The listing builds one solid part. Answer for the finished solid, in the listing's coordinates (mm). Face numbers are marked on the shaded views. A direction names the side the tool comes from. Give positions to 0.01 mm unless a question says otherwise; leave off trailing zeros. Write each loop counter-clockwise with the first axis right and the second up, starting at its lowest first coordinate (ties: lowest second). Pieces come first, ordered by that corner, then holes. Notation, with made-up numbers: (77, 46.5) - (93, 46.5) arc R17 ccw to (93, 79.5) - close; hole circle Ø3 at (-34, -5). An arc over 180 degrees is marked (long way). One line per question, with ' | ' between items. Start each with the question number.
1. A cutting plane is placed at A-A (z = 3). Determine the outline of the cut face in (x, y).
2. A cutting plane is placed at C-C (y = 27.25). Determine the outline of the cut face in (x, z), then the cut area to 3 significant figures.
3. A cutting plane is placed at D-D (z = -6.25). Determine the outline of the cut face in (x, y).
4. For the marked faces 4 and 5, determine the directions among +Z, -Z, +X, -X, +Y, -Y from which every point of the face is accessible in a straight line to the end or side of a thin tool.
5. The mould has two halves that part along Y. Classify the marked faces 1, 2 and 3: +Y half, -Y half, draft (parallel to the pull), parting line (faces both ways), or undercut.
6. A cutting plane is placed at B-B (x = 7.5). Determine the outline of the cut face in (y, z), then the cut area to 3 significant figures.
7. Given P1, Ø8.5, axis at x = -3, y = 21.5, coming from the +Z side; P2, Ø4, axis at x = 7, z = 6, coming from the +Y side, each flat-ended and moving along its own axis, determine where each tip first touches the part or whether it passes through.
8. Find the intervals of material crossed by L1, parallel to Y at x = 0, z = -8.3; L2, parallel to Z at x = 5, y = 9.5; L3, parallel to Y at x = 10, z = -3, in increasing order. Write a range as from..to.
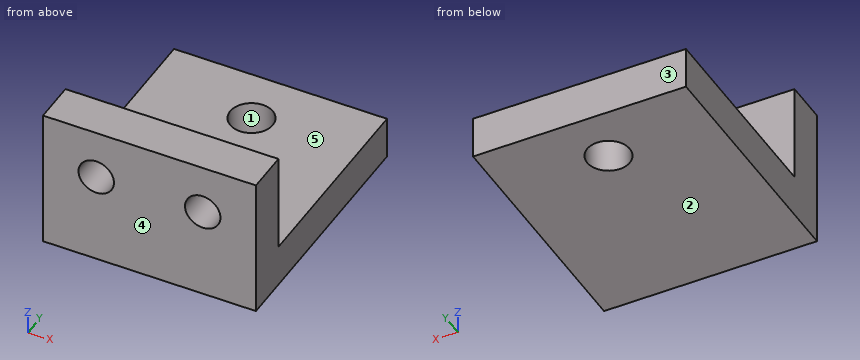
```python
from build123d import *

# Parameters (mm, degrees)
CROQUIS1_W              = 30
CROQUIS1_H              = 20
SALIENTE_EXTRUIR1_DEPTH = 6
CROQUIS2_W              = 30
CROQUIS2_H              = 35
SALIENTE_EXTRUIR2_DEPTH = 6
CROQUIS3_R              = 3
CORTAR_EXTRUIR1_DEPTH   = 6
CROQUIS4_R              = 2.5
CORTAR_EXTRUIR2_DEPTH   = 6


with BuildPart() as part:
    # Croquis1 → Saliente-Extruir1 (new body)
    with BuildSketch(Plane(origin=(0, 0, 0), x_dir=(1, 0, 0), z_dir=(0, 1, 0))):
        Rectangle(CROQUIS1_W, CROQUIS1_H)
    extrude(amount=SALIENTE_EXTRUIR1_DEPTH)

    # Croquis2 → Saliente-Extruir2 (add)
    with BuildSketch(Plane(origin=(0, 0, -10), x_dir=(-1, 0, 0), z_dir=(0, 0, -1))):
        with Locations((0, 17.5)):
            Rectangle(CROQUIS2_W, CROQUIS2_H)
    extrude(amount=-SALIENTE_EXTRUIR2_DEPTH)

    # Croquis3 → Cortar-Extruir1 (cut)
    with BuildSketch(Plane.XY.offset(-4)):
        with Locations((0, 27.25)):
            Circle(CROQUIS3_R)
    extrude(amount=-CORTAR_EXTRUIR1_DEPTH, mode=Mode.SUBTRACT)

    # Croquis4 → Cortar-Extruir2 (cut)
    with BuildSketch(Plane(origin=(0, 6, 0), x_dir=(1, 0, 0), z_dir=(0, 1, 0))):
        with Locations(Location((-7.5, -3, 0), (0, 0, 270))):
            Circle(CROQUIS4_R)
        with Locations(Location((7.5, -3, 0), (0, 0, 270))):
            Circle(CROQUIS4_R)
    extrude(amount=-CORTAR_EXTRUIR2_DEPTH, mode=Mode.SUBTRACT)


solid = part.part
```
Determined:
1) outline: (-15, 0) - (-10, 0) - (-10, 6) - (-15, 6) - close; (-5, 0) - (5, 0) - (5, 6) - (-5, 6) - close; (10, 0) - (15, 0) - (15, 6) - (10, 6) - close
2) outline: (-15, -10) - (-3, -10) - (-3, -4) - (-15, -4) - close; (3, -10) - (15, -10) - (15, -4) - (3, -4) - close | area: 144 mm2
3) outline: (-15, 0) - (15, 0) - (15, 35) - (-15, 35) - close; hole circle Ø6 at (0, 27.25)
4) face 4: +Z, -Z, +X, -X, -Y | face 5: +Z, +X, -X, +Y
5) face 1: undercut | face 2: draft | face 3: +Y half
6) outline: (0, -10) - (35, -10) - (35, -4) - (6, -4) - (6, 0.5) - (0, 0.5) - close; (0, 5.5) - (6, 5.5) - (6, 10) - (0, 10) - close | area: 264 mm2
7) P1: z = -4 | P2: y = 6
8) L1: 0..24.25, 30.25..35 | L2: -10..-4 | L3: 0..6
